from build123d import *
from OCP.BRepAlgoAPI import BRepAlgoAPI_Cut
from OCP.TopTools import TopTools_ListOfShape

# Parameters (mm, degrees)
SKETCH1_W           = 78.232
SKETCH1_H           = 90.17
BOSS_EXTRUDE1_DEPTH = 3.175
FILLET1_R           = 3.175
SKETCH2_W           = 2.032
SKETCH2_H           = 50.8
SKETCH2_W_2         = 38.1
SKETCH2_H_2         = 2.032
BOSS_EXTRUDE2_DEPTH = 5.08
FILLET3_R           = 0.508
CUT_EXTRUDE1_DEPTH  = 63.761267046
CHAMFER2_SIZE       = 0.762


with BuildPart() as part:
    # Sketch1 → Boss-Extrude1 (new body)
    with BuildSketch(Plane(origin=(0, 0, 0), x_dir=(1, 0, 0), z_dir=(0, 1, 0))):
        Rectangle(SKETCH1_W, SKETCH1_H)
        with BuildLine():
            Line((-12.319, 7.493), (12.319, 7.493))
            ThreePointArc((12.319, 7.493), (14.487025612, 8.391025612), (13.589, 6.223))
            Line((13.589, 6.223), (13.589, -6.096))
            ThreePointArc((13.589, -6.096), (14.487025612, -8.264025612), (12.319, -7.366))
            Line((12.319, -7.366), (-12.319, -7.366))
            ThreePointArc((-12.319, -7.366), (-14.487025612, -8.264025612), (-13.589, -6.096))
            Line((-13.589, -6.096), (-13.589, 6.223))
            ThreePointArc((-13.589, 6.223), (-14.487025612, 8.391025612), (-12.319, 7.493))
        make_face(mode=Mode.SUBTRACT)
    extrude(amount=BOSS_EXTRUDE1_DEPTH)

    # Fillet1
    fillet1_edges = [part.edges().sort_by_distance(p)[0] for p in [
        (-39.116, 1.5875, -45.085),
        (39.116, 1.5875, -45.085),
        (39.116, 1.5875, 45.085),
        (-39.116, 1.5875, 45.085),
    ]]
    fillet(fillet1_edges, radius=FILLET1_R)


with BuildPart() as boss_extrude2_tool:
    # Sketch2 → Boss-Extrude2 (new body)
    with BuildSketch(Plane(origin=(0, 3.175, 0), x_dir=(1, 0, 0), z_dir=(0, 1, 0))):
        Polygon((19.049995564, -47.117005476), (19.049995755, -45.085005476), (-19.050004245, -45.085001889), (-19.050004436, -47.117001889), align=None)
        with Locations((-40.132001661, 0)):
            Rectangle(SKETCH2_W, SKETCH2_H)
        with Locations((0, 46.101)):
            Rectangle(SKETCH2_W_2, SKETCH2_H_2)
        with Locations((40.132001661, 0)):
            Rectangle(SKETCH2_W, SKETCH2_H)
    extrude(amount=-BOSS_EXTRUDE2_DEPTH)


with BuildPart() as part_1:
    add(part.part)


with BuildPart() as part_2:
    # Boss-Extrude2: joined with boss_extrude2_tool
    add(part_1.part.fuse(boss_extrude2_tool.part, tol=0.00001))

    # Fillet3
    fillet3_edges = [part_2.edges().sort_by_distance(p)[0] for p in [
        (19.05, 1.5875, -45.085),
        (-19.05, 1.5875, -45.085),
        (-19.05, 0.635, -47.117),
        (19.05, 0.635, -47.117),
        (-39.116001661, 1.5875, 25.4),
        (-39.116001661, 1.5875, -25.4),
        (-41.148001661, 0.635, 25.4),
        (-41.148001661, 0.635, -25.4),
        (39.116001661, 1.5875, 25.4),
        (39.116001661, 1.5875, -25.4),
        (41.148001661, 0.635, -25.4),
        (41.148001661, 0.635, 25.4),
        (19.049995755, 1.5875, 45.085005476),
        (-19.050004245, 1.5875, 45.085001889),
        (19.049995564, 0.635, 47.117005476),
        (-19.050004436, 0.635, 47.117001889),
    ]]
    fillet(fillet3_edges, radius=FILLET3_R)


with BuildPart() as cut_extrude1_tool:
    # Sketch3 → Cut-Extrude1 (new, through all)
    with BuildSketch(Plane(origin=(0, 3.175, 0), x_dir=(1, 0, 0), z_dir=(0, 1, 0))):
        with BuildLine():
            Line((-39.116, 36.5), (-39.116, 33.5))
            ThreePointArc((-39.116, 33.5), (-37.616, 35), (-39.116, 36.5))
        make_face()
        with BuildLine():
            Line((-27.5, 45.085), (-30.5, 45.085))
            ThreePointArc((-30.5, 45.085), (-29, 43.585), (-27.5, 45.085))
        make_face()
        with BuildLine():
            Line((27.499999809, 45.084997268), (30.499999809, 45.084997268))
            ThreePointArc((30.499999809, 45.084997268), (28.999999809, 43.584997268), (27.499999809, 45.084997268))
        make_face()
        with BuildLine():
            Line((39.115998859, 36.499996315), (39.115998859, 33.499996315))
            ThreePointArc((39.115998859, 33.499996315), (37.615998859, 34.999996315), (39.115998859, 36.499996315))
        make_face()
        with BuildLine():
            Line((39.115998859, -33.499996315), (39.115998859, -36.499996315))
            ThreePointArc((39.115998859, -36.499996315), (37.615998859, -34.999996315), (39.115998859, -33.499996315))
        make_face()
        with BuildLine():
            Line((30.499999809, -45.084997268), (27.499999809, -45.084997268))
            ThreePointArc((27.499999809, -45.084997268), (28.999999809, -43.584997268), (30.499999809, -45.084997268))
        make_face()
        with BuildLine():
            Line((-27.5, -45.085), (-30.5, -45.085))
            ThreePointArc((-30.5, -45.085), (-29, -43.585), (-27.5, -45.085))
        make_face()
        with BuildLine():
            Line((-39.116, -36.5), (-39.116, -33.5))
            ThreePointArc((-39.116, -33.5), (-37.616, -35), (-39.116, -36.5))
        make_face()
    extrude(amount=-CUT_EXTRUDE1_DEPTH)


with BuildPart() as part_3:
    add(part_2.part)

    # Cut-Extrude1: cut by cut_extrude1_tool, with a tolerance
    cut_extrude1_stock = TopTools_ListOfShape()
    cut_extrude1_stock.Append(part_3.part.wrapped)
    cut_extrude1_tools = TopTools_ListOfShape()
    cut_extrude1_tools.Append(cut_extrude1_tool.part.wrapped)
    cut_extrude1_cut = BRepAlgoAPI_Cut()
    cut_extrude1_cut.SetArguments(cut_extrude1_stock)
    cut_extrude1_cut.SetTools(cut_extrude1_tools)
    cut_extrude1_cut.SetFuzzyValue(0.00001)
    cut_extrude1_cut.Build()
    add(Compound.cast(cut_extrude1_cut.Shape()).solids(), mode=Mode.REPLACE)

    # Chamfer2
    chamfer2_edges = [part_3.edges().sort_by_distance(p)[0] for p in [
        (-14.487025612, 3.175, -8.391025612),
        (-13.589, 3.175, -0.0635),
        (-14.487025612, 3.175, 8.264025612),
        (0, 3.175, 7.366),
        (14.487025612, 3.175, 8.264025612),
        (13.589, 3.175, -0.0635),
        (14.487025612, 3.175, -8.391025612),
        (0, 3.175, -7.493),
    ]]
    chamfer(chamfer2_edges, length=CHAMFER2_SIZE)


solid = part_3.part
Design review of the part built by this model. Coordinates are the model's own, in mm. A direction names the side the tool comes from. Round coordinates to 2 decimals unless told otherwise and drop trailing zeros. Write each loop counter-clockwise with the first axis right and the second up, starting at its lowest first coordinate (ties: lowest second). Pieces come first, ordered by that corner, then holes. Notation, with made-up numbers: (-31, 10) -> (5, 10) arc R17 cw to (5, 27) -> close; hole circle Ø4 at (85.5, 79). An arc over 180 degrees is marked (long way). One line per item, written item: value. Start each with the question number.
Q1. Add section C-C (x = -22). Give the boundary of the cut face in (y, z) (3 decimals).
Q2. Add section B-B (z = 16). Give the boundary of the cut face in (x, y) (3 decimals), then the cut area to 3 significant figures.
Q3. Add section A-A (z = 4). Give the boundary of the cut face in (x, y) (3 decimals).
Q4. Add section D-D (z = 35). Give the boundary of the cut face in (x, y) (3 decimals), then the cut area to 3 significant figures.
Q5. Tool access review of faces 4 (the face through (-13.589, 1, 0)), 5 (the face through (-24, 2, -45.085)), 6 (the face through (-39.116, 2, 39)), 7 (the face through (-39.116, -1, 0)): name each direction out of +Z, -Z, +X, -X, +Y, -Y from which nothing blocks a thin tool from reaching the whole face with its end or side.
Q6. To check wall thickness, follow probe 1 along X at (y, z) = (-0.85, 21.5); probe 2 along Z at (x, y) = (-3, 1.15); probe 3 along X at (y, z) = (0.85, 5.5). State the ranges of each line that lie inside material, in increasing order.
Q7. Insertion check: P1, Ø2.5, axis at x = 23.5, y = 1.5, coming from the -Z side (3 decimals); P2, Ø3.5, axis at x = -13.589, z = -7.493, coming from the -Y side; P3, Ø2, axis at x = -27.5, y = 2, coming from the +Z side (3 decimals). Each pin has a flat end and moves straight along its axis. Give the tip position at first contact, or say it passes through.
Q8. The part is to be moulded in two halves that separate along Z. For faces 1 (the face through (-38.21, 1.61, -44.13)), 2 (the face through (-29.033, 1.61, 43.585)), 3 (the face through (13.589, 1, 0)), say which applies: pulls with the +Z half, pulls with the -Z half, needs draft (parallel to the pull), parting line crosses it, or undercut.
Response:
1. outline: (0, -45.085) -> (3.175, -45.085) -> (3.175, 45.085) -> (0, 45.085) -> close
2. outline: (-41.148, -1.905) -> (-39.116, -1.905) -> (-39.116, 0) -> (39.116, 0) -> (39.116, -1.905) -> (41.148, -1.905) -> (41.148, 3.175) -> (-41.148, 3.175) -> close
2. area: 269 mm^2
3. outline: (-41.148, -1.905) -> (-39.116, -1.905) -> (-39.116, 0) -> (-13.589, 0) -> (-13.589, 2.413) -> (-14.351, 3.175) -> (-41.148, 3.175) -> close; (13.589, 0) -> (39.116, 0) -> (39.116, -1.905) -> (41.148, -1.905) -> (41.148, 3.175) -> (14.351, 3.175) -> (13.589, 2.413) -> close
4. outline: (-37.616, 0) -> (37.616, 0) -> (37.616, 3.175) -> (-37.616, 3.175) -> close
4. area: 239 mm^2
5. face 4: +Y, -Y
5. face 5: -Z, -X, +Y, -Y
5. face 6: +Z, -X, +Y, -Y
5. face 7: +Z, -Z, -Y
6. probe 1: x = -41.15 to -39.12, 39.12 to 41.15
6. probe 2: z = -47.12 to -7.49, 7.37 to 47.12
6. probe 3: x = -41.15 to -13.59, 13.59 to 41.15
7. P1: stops at z = -45.085
7. P2: stops at y = 0
7. P3: stops at z = 45.085
8. face 1: pulls with the -Z half
8. face 2: pulls with the +Z half
8. face 3: undercut
